Read the model definition and answer for the solid it produces. Units are mm, in the model's axes. A direction names the side the tool comes from. Coordinates: 2 decimals unless noted, no trailing zeros. Order: outer loops, then holes, each group sorted by start corner. A loop starts at its lowest first (then second) coordinate and runs counter-clockwise, first axis right, second up.
```python
from build123d import *

# Parameters (mm, degrees)
SKETCH1_W           = 58.1
SKETCH1_H           = 40.11
BOSS_EXTRUDE1_DEPTH = 27
SKETCH2_R           = 9.5
BOSS_EXTRUDE2_DEPTH = 2
SKETCH3_R           = 4
BOSS_EXTRUDE3_DEPTH = 15
SKETCH4_W           = 6.276876118
SKETCH4_H           = 1.998885949
CUT_EXTRUDE1_DEPTH  = 13
SKETCH5_R           = 3
BOSS_EXTRUDE4_DEPTH = 2
SKETCH6_R           = 2
CUT_EXTRUDE2_DEPTH  = 8
SKETCH7_R           = 4
CUT_EXTRUDE3_DEPTH  = 25.4


with BuildPart() as part:
    # Sketch1 → Boss-Extrude1 (new body)
    with BuildSketch(Plane.XY):
        with Locations((29.05, 20.055)):
            Rectangle(SKETCH1_W, SKETCH1_H)
    extrude(amount=BOSS_EXTRUDE1_DEPTH)

    # Sketch2 → Boss-Extrude2 (add)
    with BuildSketch(Plane.XY.offset(27)):
        with Locations((20.2, 20.055)):
            Circle(SKETCH2_R)
    extrude(amount=BOSS_EXTRUDE2_DEPTH)

    # Sketch3 → Boss-Extrude3 (add)
    with BuildSketch(Plane.XY.offset(29)):
        with Locations((20.2, 20.055)):
            Circle(SKETCH3_R)
    extrude(amount=BOSS_EXTRUDE3_DEPTH)

    # Sketch4 → Cut-Extrude1 (cut)
    with BuildSketch(Plane.XY.offset(44)):
        with Locations((20.2, 23.534403972)):
            Rectangle(SKETCH4_W, SKETCH4_H)
    extrude(amount=-CUT_EXTRUDE1_DEPTH, mode=Mode.SUBTRACT)

    # Sketch5 → Boss-Extrude4 (add)
    with BuildSketch(Plane.XY.offset(27)):
        with Locations((9.05, 34.055)):
            Circle(SKETCH5_R)
        with Locations((49.05, 34.055)):
            Circle(SKETCH5_R)
        with Locations((49.05, 6.055)):
            Circle(SKETCH5_R)
        with Locations((9.05, 6.055)):
            Circle(SKETCH5_R)
    extrude(amount=BOSS_EXTRUDE4_DEPTH)

    # Sketch6 → Cut-Extrude2 (cut)
    with BuildSketch(Plane.XY.offset(29)):
        with Locations((9.05, 34.055)):
            Circle(SKETCH6_R)
        with Locations((49.05, 34.055)):
            Circle(SKETCH6_R)
        with Locations((49.05, 6.055)):
            Circle(SKETCH6_R)
        with Locations((9.05, 6.055)):
            Circle(SKETCH6_R)
    extrude(amount=-CUT_EXTRUDE2_DEPTH, mode=Mode.SUBTRACT)

    # Sketch7 → Cut-Extrude3 (cut)
    with BuildSketch(Plane(origin=(58.1, 0, 0), x_dir=(0, 0, -1), z_dir=(1, 0, 0))):
        with Locations((-15.797911108, 20)):
            Circle(SKETCH7_R)
    extrude(amount=-CUT_EXTRUDE3_DEPTH, mode=Mode.SUBTRACT)


solid = part.part
```
1) A cutting plane is placed at D-D, the plane y = 13. Determine the outline of the cut face in (x, z), and give its area (3 significant figures).
A:
outline: (0, 0) - (58.1, 0) - (58.1, 27) - (26.56, 27) - (26.56, 29) - (13.84, 29) - (13.84, 27) - (0, 27) - close
area: 1,590 mm2
2) Flat-ended cylindrical pins translate along their axes: pin 1 Ø3 at (x, y) = (9.05, 6.055) entering from -Z; pin 2 Ø7 at (x, z) = (19, 36.5) entering from +Y; pin 3 Ø1.2 at (x, y) = (9, 33.5) entering from +Z; pin 4 Ø8 at (x, y) = (43, 9.5) entering from +Z. Find the tip coordinate at first contact, or state that the pin passes through.
A:
pin 1: stops at z = 0
pin 2: stops at y = 22.53
pin 3: stops at z = 21
pin 4: stops at z = 29
3) Determine the mould class of faces 6 (the flat face through (9, 6, 21)), 7 (the flat face through (29, 40.11, 13)), 8 (the flat face through (49, 6, 21)), 9 (the flat face through (51, 5, 29)) for opening direction Y: pulls with the +Y half, pulls with the -Y half, needs draft (parallel to the pull), parting line crosses it, or undercut.
A:
face 6: undercut
face 7: pulls with the +Y half
face 8: undercut
face 9: needs draft
4) Which of the six approach directions +Z, -Z, +X, -X, +Y, -Y give full straight-line access (tool end or side, diameter ignored) to faces 1 (the flat face through (20, 22.535, 38)), 2 (the flat face through (10, 4, 29)), 3 (the flat face through (29, 0, 13)), 4 (the cylindrical face through (50.958, 34.656, 25.056)), 5 (the cylindrical face through (45.578, 21.201, 11.983))?
A:
face 1: +Z, +X, -X, +Y
face 2: +Z, +X, -X, +Y, -Y
face 3: +Z, -Z, +X, -X, -Y
face 4: +Z
face 5: +X
5) A cutting plane is placed at A-A, the plane x = 9.05. Determine the outline of the cut face in (y, z) (3 decimals).
A:
outline: (0, 0) - (40.11, 0) - (40.11, 27) - (37.055, 27) - (37.055, 29) - (36.055, 29) - (36.055, 21) - (32.055, 21) - (32.055, 29) - (31.055, 29) - (31.055, 27) - (9.055, 27) - (9.055, 29) - (8.055, 29) - (8.055, 21) - (4.055, 21) - (4.055, 29) - (3.055, 29) - (3.055, 27) - (0, 27) - close
6) Straight lines are drawn through the part: line 1 (Y direction, x = 49.05, z = 25.25) (3 decimals); line 2 (X direction, y = 6, z = 24); line 3 (Z direction, x = 20, y = 35.5). For each, find the intervals that lie inside material, in ascending order.
A:
line 1: y = 0 to 4.055, 8.055 to 32.055, 36.055 to 40.11
line 2: x = 0 to 7.05, 11.05 to 47.05, 51.05 to 58.1
line 3: z = 0 to 27
7) A cutting plane is placed at C-C, the plane z = 13. Determine the outline of the cut face in (x, y), and give its area (3 significant figures).
A:
outline: (0, 0) - (58.1, 0) - (58.1, 17.14) - (32.7, 17.14) - (32.7, 22.86) - (58.1, 22.86) - (58.1, 40.11) - (0, 40.11) - close
area: 2,190 mm2
8) A cutting plane is placed at B-B, the plane x = 42.5. Determine the outline of the cut face in (y, z), and give its area (3 significant figures).
A:
outline: (0, 0) - (40.11, 0) - (40.11, 27) - (0, 27) - close; hole circle Ø8 at (20, 15.8)
area: 1,030 mm2
